from build123d import *

# Parameters (mm, degrees)
SKETCH2_R           = 12
BOSS_EXTRUDE1_DEPTH = 10
BOSS_EXTRUDE2_DEPTH = 3
SKETCH4_W           = 20
SKETCH4_H           = 2
BOSS_EXTRUDE3_DEPTH = 60
SKETCH5_R           = 10
CUT_EXTRUDE1_DEPTH  = 8


with BuildPart() as part:
    # Sketch2 → Boss-Extrude1 (new body)
    with BuildSketch(Plane.XY):
        Circle(SKETCH2_R)
    extrude(amount=BOSS_EXTRUDE1_DEPTH)

    # Sketch3 → Boss-Extrude2 (add)
    with BuildSketch(Plane.XY.offset(10)):
        with BuildLine():
            Line((-10, -26), (-10, -6.633249581))
            ThreePointArc((-10, -6.633249581), (0, -12), (10, -6.633249581))
            Line((10, -6.633249581), (10, -26))
            Line((10, -26), (-10, -26))
        make_face()
    extrude(amount=-BOSS_EXTRUDE2_DEPTH)

    # Sketch4 → Boss-Extrude3 (add)
    with BuildSketch(Plane.XY.offset(10)):
        with Locations((0, -25)):
            Rectangle(SKETCH4_W, SKETCH4_H)
    extrude(amount=BOSS_EXTRUDE3_DEPTH)

    # Sketch5 → Cut-Extrude1 (cut)
    with BuildSketch(Plane(origin=(0, 0, 0), x_dir=(-1, 0, 0), z_dir=(0, 0, -1))):
        Circle(SKETCH5_R)
    extrude(amount=-CUT_EXTRUDE1_DEPTH, mode=Mode.SUBTRACT)


solid = part.part
Build history of the part. All positions in model axes, mm. A direction names the side the tool comes from. Round coordinates to 2 decimals unless told otherwise and drop trailing zeros. Write each loop counter-clockwise with the first axis right and the second up, starting at its lowest first coordinate (ties: lowest second). Pieces come first, ordered by that corner, then holes. Notation, with made-up numbers: M 3.5,37 L 8.5,37 A15 cw 8.5,55 Z; hole C 86.5,31 d10. An arc over 180 degrees is marked long. Answer in a Markdown table with one row per item.
1. Flat gauge pins, fed straight in: P1, Ø6, axis at x = 4, y = -2.5, coming from the -Z side; P2, Ø1.5, axis at x = -8, y = -18, coming from the -Z side; P3, Ø1, axis at x = 3, y = -6.5, coming from the +Z side. Where does each tip first touch, or does it go through?
Geometry check:
| item | result |
|---|---|
| P1 | z = 8 |
| P2 | z = 7 |
| P3 | z = 10 |
2. Saw through at C-C (z = 59.5). List the corners of the cut face in (x, y), and give its area (3 significant figures).
Geometry check:
| item | result |
|---|---|
| outline | M -10,-26 L 10,-26 L 10,-24 L -10,-24 Z |
| area | 40.0 mm2 |
3. Saw through at B-B (y = 0). List the corners of the cut face in (x, z), and give its area (3 significant figures).
Geometry check:
| item | result |
|---|---|
| outline | M -12,0 L -10,0 L -10,8 L 10,8 L 10,0 L 12,0 L 12,10 L -12,10 Z |
| area | 80.0 mm2 |
4. Saw through at A-A (x = 0). List the corners of the cut face in (y, z), and give its area (3 significant figures).
Geometry check:
| item | result |
|---|---|
| outline | M -26,7 L -12,7 L -12,0 L -10,0 L -10,8 L 10,8 L 10,0 L 12,0 L 12,10 L -24,10 L -24,70 L -26,70 Z |
| area | 242 mm2 |
5. Mould opens along Y. For faces 1 (the face through (2.17, -9.76, 3.94)), 2 (the face through (0, 0, 8)), 3 (the face through (0, -25, 70)), 4 (the face through (0, -26, 38)) say: +Y half, -Y half, draft (parallel to the pull), parting line (faces both ways), or undercut.
Geometry check:
| item | result |
|---|---|
| face 1 | undercut |
| face 2 | undercut |
| face 3 | draft |
| face 4 | -Y half |
6. Which spindle directions (+Z, -Z, +X, -X, +Y, -Y) get a long thin tool onto all of the face, cutting with end or side? Do faces 5 (the face through (-10, -24.3, 31.4)), 6 (the face through (0, -24, 40)), 7 (the face through (10, -24.3, 31.4)). Say none if no direction does.
Geometry check:
| item | result |
|---|---|
| face 5 | +Z, -Z, -X, -Y |
| face 6 | +Z, +X, -X, +Y |
| face 7 | +Z, -Z, +X, -Y |
7. Saw through at D-D (x = 6.75). List the corners of the cut face in (y, z), and give its area (3 significant figures).
Geometry check:
| item | result |
|---|---|
| outline | M -26,7 L -9.92,7 L -9.92,0 L -7.38,0 L -7.38,8 L 7.38,8 L 7.38,0 L 9.92,0 L 9.92,10 L -24,10 L -24,70 L -26,70 Z |
| area | 249 mm2 |
8. Probe L1, parallel to Y at x = 0, z = 4.75; L2, parallel to Y at x = -1.75, z = 38; L3, parallel to Z at x = 6.75, y = -14. List the from-to ranges inside material, lowest first. Write a range as [from, to].
Geometry check:
| item | result |
|---|---|
| L1 | [-12, -10], [10, 12] |
| L2 | [-26, -24] |
| L3 | [7, 10] |
